from build123d import *

# Parameters (mm, degrees)
SKETCH_1_R               = 15
SKETCH_1_R_2             = 2
SKETCH_1_R_3             = 1.5
EXTRUDE_1_DEPTH          = 3
EXTRUDE_2_DEPTH          = 4.25
EXTRUDE_2_DEPTH_BACK     = 7.25
SKETCH_2_R               = 8
EXTRUDE_3_DEPTH          = 1.25
EXTRUDE_3_DEPTH_BACK     = 4.25
SKETCH_5_R               = 15
CUT_EXTRUDE_1_DEPTH      = 5
CUT_EXTRUDE_1_DEPTH_BACK = 16.5
SKETCH_3_R               = 2.5
SKETCH_7_R               = 1.5
CUT_EXTRUDE_4_DEPTH      = 14
SKETCH_9_R               = 5
CUT_EXTRUDE_6_DEPTH      = 5


with BuildPart() as part:
    # 草图1 → 凸台-拉伸1 (new body)
    with BuildSketch(Plane(origin=(0, 0, 0), x_dir=(1, 0, 0), z_dir=(0, 1, 0))):
        with Locations(Location((0, 0, 0), (0, 0, 270))):
            Circle(SKETCH_1_R)
        with Locations(Location((0, 0, 0), (0, 0, 270))):
            Circle(SKETCH_1_R_2, mode=Mode.SUBTRACT)
        with Locations(Location((0, 6, 0), (0, 0, 270))):
            Circle(SKETCH_1_R_3, mode=Mode.SUBTRACT)
        with Locations(Location((6, 0, 0), (0, 0, 270))):
            Circle(SKETCH_1_R_3, mode=Mode.SUBTRACT)
        with Locations(Location((0, -6, 0), (0, 0, 270))):
            Circle(SKETCH_1_R_3, mode=Mode.SUBTRACT)
        with Locations(Location((-6, 0, 0), (0, 0, 270))):
            Circle(SKETCH_1_R_3, mode=Mode.SUBTRACT)
        with Locations(Location((0, 12, 0), (0, 0, 270))):
            Circle(SKETCH_1_R_3, mode=Mode.SUBTRACT)
        with Locations(Location((12, 0, 0), (0, 0, 270))):
            Circle(SKETCH_1_R_3, mode=Mode.SUBTRACT)
        with Locations(Location((0, -12, 0), (0, 0, 270))):
            Circle(SKETCH_1_R_3, mode=Mode.SUBTRACT)
        with Locations(Location((-12, 0, 0), (0, 0, 270))):
            Circle(SKETCH_1_R_3, mode=Mode.SUBTRACT)
    extrude(amount=EXTRUDE_1_DEPTH)

    # 草图2 → 凸台-拉伸2 (add, two sides: drawn at the far end of the back side and taken through both)
    with BuildSketch(Plane.XZ.offset(-EXTRUDE_2_DEPTH_BACK)):
        with Locations(Location((0, 0, 0), (0, 0, 270))):
            Circle(SKETCH_2_R)
    extrude(amount=EXTRUDE_2_DEPTH + EXTRUDE_2_DEPTH_BACK)

    # 草图5 → 凸台-拉伸3 (add, two sides: drawn at the far end of the back side and taken through both)
    with BuildSketch(Plane(origin=(0, 3, 0), x_dir=(1, 0, 0), z_dir=(0, 1, 0)).offset(-EXTRUDE_3_DEPTH_BACK)):
        with Locations(Location((0, 0, 0), (0, 0, 270))):
            Circle(SKETCH_5_R)
    extrude(amount=EXTRUDE_3_DEPTH + EXTRUDE_3_DEPTH_BACK)

    # 草图3 → 切除-拉伸1 (cut, two sides: drawn at the far end of the back side and taken through both)
    with BuildSketch(Plane(origin=(0, 3, 0), x_dir=(1, 0, 0), z_dir=(0, 1, 0)).offset(-CUT_EXTRUDE_1_DEPTH_BACK)):
        with Locations(Location((0, 0, 0), (0, 0, 90))):
            Circle(SKETCH_3_R)
    extrude(amount=CUT_EXTRUDE_1_DEPTH + CUT_EXTRUDE_1_DEPTH_BACK, mode=Mode.SUBTRACT)

    # 草图7 → 切除-拉伸4 (cut)
    with BuildSketch(Plane(origin=(0, 7.25, 0), x_dir=(1, 0, 0), z_dir=(0, 1, 0))):
        with Locations(Location((0, 12, 0), (0, 0, 270))):
            Circle(SKETCH_7_R)
        with Locations(Location((-12, 0, 0), (0, 0, 270))):
            Circle(SKETCH_7_R)
        with Locations(Location((12, 0, 0), (0, 0, 270))):
            Circle(SKETCH_7_R)
        with Locations(Location((0, -12, 0), (0, 0, 270))):
            Circle(SKETCH_7_R)
    extrude(amount=-CUT_EXTRUDE_4_DEPTH, mode=Mode.SUBTRACT)

    # 草图9 → 切除-拉伸6 (cut)
    with BuildSketch(Plane.XZ.offset(4.25)):
        with Locations(Location((0, 0, 0), (0, 0, 270))):
            Circle(SKETCH_9_R)
    extrude(amount=-CUT_EXTRUDE_6_DEPTH, mode=Mode.SUBTRACT)


solid = part.part
Geometry: final body of the model. Coordinates: model frame, mm. A direction names the side the tool comes from. Give positions to 0.01 mm unless a question says otherwise; leave off trailing zeros. Write each loop counter-clockwise with the first axis right and the second up, starting at its lowest first coordinate (ties: lowest second). Pieces come first, ordered by that corner, then holes.
(1) Cut plane B-B, the plane z = -12. Return loops of the section in (x, y), then the cut area to 3 significant figures.
(2) Cut plane C-C, the plane y = 3.5. Return loops of the section in (x, z).
(3) Access query for faces 1 (the flat face through (-6, 4.25, 6)), 2 (the cylindrical face through (-7.81, -2.73, 1.73)), 3 (the cylindrical face through (0.07, 1.54, 10.5)). Directions: +Z, -Z, +X, -X, +Y, -Y. A direction counts if a zero-diameter tool reaches every point of the face in a straight line with its end or side. Return the directions, or none.
(4) First-contact query: P1, Ø4, axis at x = 0, z = 12, coming from the +Y side; P2, Ø1, axis at x = -9.5, z = -2, coming from the -Y side; P3, Ø1.5, axis at x = 5.5, y = 2.5, coming from the -Z side. Flat tips, straight axial feed; report the tip coordinate or a pass-through.
(5) Ray query, line 1 (X direction, y = 1.15, z = 0); line 2 (X direction, y = -2.5, z = 0); line 3 (X direction, y = -0.5, z = 1). Return the intervals inside material, ascending.
(6) Cut plane D-D, the plane z = -0.25. Return loops of the section in (x, y), then the cut area to 3 significant figures.
(7) Cut plane A-A, the plane x = 12. Return loops of the section in (y, z), then the cut area to 3 significant figures.
(8) Mould query, pull axis X, two halves, no side actions, for faces 4 (the cylindrical face through (12.45, 1.54, 1.43)), 5 (the cylindrical face through (-7.81, 5.77, 1.73)), 6 (the flat face through (-6, -1.25, 6)). Classes: released by +X, released by -X, zero draft, split by the parting line, or undercut.
Values follow:
1. outline: (-9, -1.25) - (-1.5, -1.25) - (-1.5, 4.25) - (-9, 4.25) - close; (1.5, -1.25) - (9, -1.25) - (9, 4.25) - (1.5, 4.25) - close
1. area: 82.5 mm2
2. outline: circle Ø30 at (0, 0); hole circle Ø3 at (-12, 0); hole circle Ø5 at (0, 0); hole circle Ø3 at (0, -12); hole circle Ø3 at (0, 12); hole circle Ø3 at (12, 0)
3. face 1: +Y
3. face 2: -Y
3. face 3: +Y, -Y
4. P1: stops at y = 4.25
4. P2: stops at y = -1.25
4. P3: stops at z = -14.23
5. line 1: x = -15 to -13.5, -10.5 to -2.5, 2.5 to 10.5, 13.5 to 15
5. line 2: x = -8 to -5, 5 to 8
5. line 3: x = -14.97 to -13.12, -10.88 to -4.9, 4.9 to 10.88, 13.12 to 14.97
6. outline: (-15, -1.25) - (-13.48, -1.25) - (-13.48, 4.25) - (-15, 4.25) - close; (-10.52, -1.25) - (-8, -1.25) - (-8, -4.25) - (-4.99, -4.25) - (-4.99, 0.75) - (-2.49, 0.75) - (-2.49, 7.25) - (-8, 7.25) - (-8, 4.25) - (-10.52, 4.25) - close; (2.49, 0.75) - (4.99, 0.75) - (4.99, -4.25) - (8, -4.25) - (8, -1.25) - (10.52, -1.25) - (10.52, 4.25) - (8, 4.25) - (8, 7.25) - (2.49, 7.25) - close; (13.48, -1.25) - (15, -1.25) - (15, 4.25) - (13.48, 4.25) - close
6. area: 146 mm2
7. outline: (-1.25, -9) - (4.25, -9) - (4.25, -1.5) - (-1.25, -1.5) - close; (-1.25, 1.5) - (4.25, 1.5) - (4.25, 9) - (-1.25, 9) - close
7. area: 82.5 mm2
8. face 4: undercut
8. face 5: split by the parting line
8. face 6: zero draft
